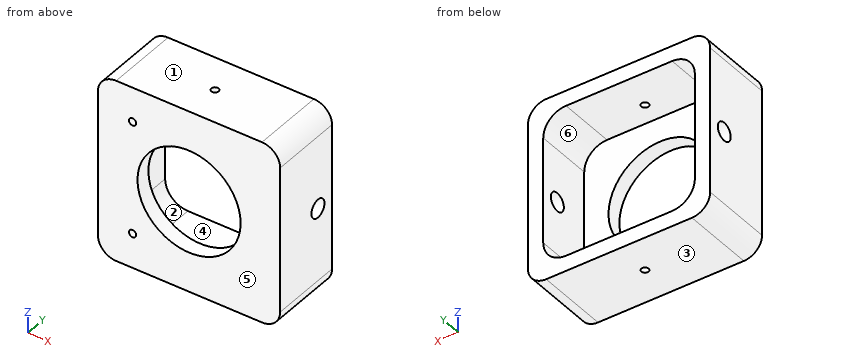
Autodesk Inventor part; units mm, degrees
ref_plane "Work Plane1" through (0, 25.4, -26.416) normal (-1, 0, 0) x (0, 0, 1)
ref_plane "YZ Plane" through (0, 0, 0) normal (1, 0, 0) x (0, 1, 0)
ref_plane "XZ Plane" through (0, 0, 0) normal (0, 1, 0) x (-1, 0, 0)
sketch "Sketch2" plane through (0, 0, 0) normal (0, 1, 0) x (-1, 0, 0)
  line L0 (-31.75, 31.75) -> (31.75, 31.75)
  line L1 (31.75, 31.75) -> (31.75, -31.75)
  line L2 (31.75, -31.75) -> (-31.75, -31.75)
  line L3 (-31.75, -31.75) -> (-31.75, 31.75)
  line L4 (-31.75, 31.75) -> (31.75, -31.75) construction
  line L5 (31.75, 31.75) -> (-31.75, -31.75) construction
  point P0 (0, 0)
  dimension "d3" = 63.5
  dimension "d4" = 63.5
extrude "Extrusion2" add sketch "Sketch2" along normal blind 25.4
fillet "Fillet1" radius 6.35 4 edges at (31.75, 12.7, 31.75) (31.75, 12.7, -31.75) (-31.75, 12.7, -31.75) (-31.75, 12.7, 31.75)
sketch "Sketch3" plane through (0, 25.4, 0) normal (0, 1, 0) x (1, 0, 0)
  arc A0 (-31.75, -25.4) -> (-25.4, -31.75) centre (-25.4, -25.4) ccw
  line L0 (-25.4, -31.75) -> (25.4, -31.75)
  arc A1 (25.4, -31.75) -> (31.75, -25.4) centre (25.4, -25.4) ccw
  line L1 (31.75, -25.4) -> (31.75, 25.4)
  arc A2 (31.75, 25.4) -> (25.4, 31.75) centre (25.4, 25.4) ccw
  line L2 (25.4, 31.75) -> (-25.4, 31.75)
  arc A3 (-25.4, 31.75) -> (-31.75, 25.4) centre (-25.4, 25.4) ccw
  line L3 (-31.75, 25.4) -> (-31.75, -25.4)
  line L4 (-26.416, 26.416) -> (26.416, 26.416)
  line L5 (26.416, 26.416) -> (26.416, -26.416)
  line L6 (26.416, -26.416) -> (-26.416, -26.416)
  line L7 (-26.416, -26.416) -> (-26.416, 26.416)
  point P0 (0, 0)
  dimension "d8" = 5.334
extrude "Extrusion3" cut sketch "Sketch3" against normal blind 20.066 contours L4 L5 L6 L7
ref_plane "Work Plane1" through (0, 25.4, -26.416) normal (-1, 0, 0) x (0, 0, 1)
fillet "Fillet2" radius 7.9375 4 edges at (-26.416, 15.367, 26.416) (-26.416, 15.367, -26.416) (26.416, 15.367, -26.416) (26.416, 15.367, 26.416)
sketch "Sketch6" plane through (-25.4, 0, 31.75) normal (0, 0, 1) x (1, 0, 0)
  line L0 (0, 0) -> (0, 25.4)
  line L1 (50.8, 0) -> (0, 0)
  line L2 (50.8, 25.4) -> (50.8, 0)
  line L3 (0, 25.4) -> (50.8, 25.4)
  circle A0 centre (25.4, 12.7) radius 1.27
  point P0 (25.4, 0)
  dimension "d31" = 2.54
  dimension "d32" = 12.7
  dimension "d33" = 25.4
hole "Hole3" at (0, 12.7, 31.75) direction (0, 0, -1) diameter 2.54 depth 76.2 tip angle 118
sketch "Sketch8" plane through (0, 0, 0) normal (0, -1, 0) x (1, 0, 0)
  point P0 (0, 0)
sketch "Sketch9" plane through (0, 0, 0) normal (0, -1, 0) x (1, 0, 0)
  line L0 (25.4, 28.575) -> (-15.875, 28.575)
  arc A0 (-15.875, 28.575) -> (-28.575, 15.875) centre (-15.875, 15.875) ccw
  line L1 (-28.575, 15.875) -> (-28.575, -15.875)
  arc A1 (-28.575, -15.875) -> (-15.875, -28.575) centre (-15.875, -15.875) ccw
  line L2 (-15.875, -28.575) -> (25.4, -28.575)
  arc A2 (25.4, -28.575) -> (28.575, -25.4) centre (25.4, -25.4) ccw
  line L3 (28.575, -25.4) -> (28.575, -1.27)
  line L4 (28.575, -1.27) -> (17.9256, -1.27)
  circle A3 centre (0, 0) radius 17.9705
  line L5 (17.9256, 1.27) -> (28.575, 1.27)
  line L6 (28.575, 1.27) -> (28.575, 25.4)
  arc A4 (28.575, 25.4) -> (25.4, 28.575) centre (25.4, 25.4) ccw
  circle A5 centre (-19.685, -19.685) radius 1.27
  circle A6 centre (-19.685, 19.685) radius 1.27
  dimension "d53" = 2.54
  dimension "d54" = 3.81
  dimension "d55" = 3.81
  dimension "d56" = 2.54
  dimension "d57" = 3.81
  dimension "d58" = 3.81
extrude "Extrusion6" cut sketch "Sketch9" against normal blind 25.4 contours A3 | A5 | A6
sketch "Sketch10" plane through (31.75, 0, 25.4) normal (1, 0, 0) x (0, 0, -1)
  circle A0 centre (25.4, 18.5) radius 3.175
  point P0 (25.4, 0)
  dimension "d61" = 6.35
extrude "Extrusion7" cut sketch "Sketch10" against normal blind 6.35
sketch "Sketch11" plane through (-31.75, 0, -25.4) normal (-1, 0, 0) x (0, 0, 1)
  circle A0 centre (25.4, 18.5) radius 3.175
  circle A1 centre (25.4, 18.5) radius 3.175
  point P0 (25.4, 0)
extrude "Extrusion8" cut sketch "Sketch11" against normal blind 25.4
properties part number "basemotor"
The model under review builds one solid part; all positions refer to its coordinate system, in mm. Face numbers are marked on the shaded views. A direction names the side the tool comes from. Round coordinates to 2 decimals unless told otherwise and drop trailing zeros. Write each loop counter-clockwise with the first axis right and the second up, starting at its lowest first coordinate (ties: lowest second). Pieces come first, ordered by that corner, then holes. Notation, with made-up numbers: (73, 76) - (83, 76) arc R11 cw to (83, 92) - close; hole circle Ø5 at (6, 52.25). An arc over 180 degrees is marked (long way). Answer as CSV lines item,"result". Start each with the question number.
(1) We need section D-D on z = 8.5. State the section outline as (x, y) points, plus the area to 3 significant figures.
(2) We need section B-B on z = 0. Give the number of separate pieces and of enclosed holes in the cut face, plus the area to 3 significant figures.
(3) To check wall thickness, follow line 1 (Z direction, x = -9.5, y = 19.5); line 2 (Z direction, x = 0, y = 1.2). State the ranges of each line that lie inside material, in increasing order.
(4) Draft analysis for pull direction Z (two halves, no side actions). For the marked faces 1, 2, 3 and 4, state which applies: pulls with the +Z half, pulls with the -Z half, needs draft (parallel to the pull), parting line crosses it, or undercut.
(5) We need section C-C on x = -13. State the section outline as (y, z) points.
(6) For pin 1 Ø3 at (x, y) = (0, 12.7) entering from +Z; pin 2 Ø5 at (y, z) = (18.5, 0) entering from -X, all flat-tipped, find the tip position at first contact; note any pin that passes through.
(7) For the marked faces 5 and 6, list the 3-axis set-ups (+Z, -Z, +X, -X, +Y, -Y) from which the entire face can be reached by the end or side of a thin tool; tool diameter is ignored.
Worked answers:
1,outline,"(-31.75, 0) - (-15.83, 0) - (-15.83, 5.33) - (-26.42, 5.33) - (-26.42, 25.4) - (-31.75, 25.4) - close; (15.83, 0) - (31.75, 0) - (31.75, 25.4) - (26.42, 25.4) - (26.42, 5.33) - (15.83, 5.33) - close"
1,area,"384 mm²"
2,separate pieces,"4"
2,enclosed holes,"0"
2,area,"293 mm²"
3,line 1,"-31.75 to -26.42, 26.42 to 31.75"
3,line 2,"-31.75 to -17.97, 17.97 to 31.75"
4,face 1,"pulls with the +Z half"
4,face 2,"undercut"
4,face 3,"pulls with the -Z half"
4,face 4,"undercut"
5,outline,"(0, -31.75) - (25.4, -31.75) - (25.4, -26.42) - (5.33, -26.42) - (5.33, -12.41) - (0, -12.41) - close; (0, 12.41) - (5.33, 12.41) - (5.33, 26.42) - (25.4, 26.42) - (25.4, 31.75) - (0, 31.75) - close"
6,pin 1,"z = 31.75"
6,pin 2,"through"
7,face 5,"+Z, -Z, +X, -X, -Y"
7,face 6,"+Y"
